Autodesk Inventor part; units mm, degrees
ref_plane "YZ Plane" through (0, 0, 0) normal (1, 0, 0) x (0, 1, 0)
ref_plane "XZ Plane" through (0, 0, 0) normal (0, 1, 0) x (-1, 0, 0)
ref_plane "XY Plane" through (0, 0, 0) normal (0, 0, 1) x (1, 0, 0)
sketch "Sketch1" plane through (0, 0, 0) normal (0, 1, 0) x (-1, 0, 0)
  line L0 (0, 0) -> (41.3, 0)
  line L1 (41.3, 0) -> (41.3, 41.3)
  line L2 (41.3, 41.3) -> (0, 41.3)
  line L3 (0, 41.3) -> (0, 0)
  dimension "d0" = 41.3
  dimension "d1" = 41.3
extrude "Extrusion1" add sketch "Sketch1" along normal blind 10
sketch "Sketch8" plane through (0, 10, 0) normal (0, 1, 0) x (1, 0, 0)
  line L0 (-1, -1) -> (-40.3, -1)
  line L1 (-40.3, -1) -> (-40.3, -40.3)
  line L2 (-40.3, -40.3) -> (-1, -40.3)
  line L3 (-1, -40.3) -> (-1, -1)
  line L4 (0, 0) -> (-41.3, 0)
  line L5 (0, -41.3) -> (0, 0)
  dimension "d61" = 39.3
  dimension "d62" = 39.3
  dimension "d63" = 1
  dimension "d64" = 1
extrude "Extrusion7" cut sketch "Sketch8" against normal blind 8.5
sketch "Sketch9" plane through (0, 1.5, 0) normal (0, 1, 0) x (1, 0, 0)
  line L0 (-3.45, -3.45) -> (-18.15, -3.45)
  line L1 (-18.15, -3.45) -> (-18.15, -18.15)
  line L2 (-18.15, -18.15) -> (-3.45, -18.15)
  line L3 (-3.45, -18.15) -> (-3.45, -3.45)
  line L4 (-1, -1) -> (-1, -40.3)
  line L5 (-40.3, -1) -> (-1, -1)
  line L6 (-23.15, -3.45) -> (-37.85, -3.45)
  line L7 (-37.85, -3.45) -> (-37.85, -18.15)
  line L8 (-37.85, -18.15) -> (-23.15, -18.15)
  line L9 (-23.15, -18.15) -> (-23.15, -3.45)
  line L10 (-23.15, -23.15) -> (-37.85, -23.15)
  line L11 (-37.85, -23.15) -> (-37.85, -37.85)
  line L12 (-37.85, -37.85) -> (-23.15, -37.85)
  line L13 (-23.15, -37.85) -> (-23.15, -23.15)
  line L14 (-40.3, -40.3) -> (-40.3, -1)
  line L15 (-18.15, -23.15) -> (-3.45, -23.15)
  line L16 (-3.45, -23.15) -> (-3.45, -37.85)
  line L17 (-3.45, -37.85) -> (-18.15, -37.85)
  line L18 (-18.15, -37.85) -> (-18.15, -23.15)
  point P0 (0, 0)
  dimension "d67" = 14.7
  dimension "d68" = 14.7
  dimension "d69" = 2.45
  dimension "d70" = 2.45
  dimension "d71" = 14.7
  dimension "d72" = 14.7
  dimension "d73" = 5
  dimension "d74" = 14.7
  dimension "d75" = 14.7
  dimension "d76" = 5
  dimension "d77" = 2.45
  dimension "d78" = 14.7
  dimension "d79" = 14.7
  dimension "d80" = 5
  dimension "d81" = 5
extrude "Extrusion8" cut sketch "Sketch9" against normal blind 8.5
properties part number "test plate"
Read the model definition and answer for the solid it produces. Units are mm, in the model's axes. A direction names the side the tool comes from. Give positions to 0.01 mm unless a question says otherwise; leave off trailing zeros. Write each loop counter-clockwise with the first axis right and the second up, starting at its lowest first coordinate (ties: lowest second). Pieces come first, ordered by that corner, then holes. Notation, with made-up numbers: (-36, 84) -> (23, 84) arc R14 cw to (23, 88) -> close; hole circle Ø6 at (17.5, -35.5). An arc over 180 degrees is marked (long way). Answer as a JSON object with one key per item and string values.
1) Straight lines are drawn through the part: probe 1 along X at (y, z) = (1, 25.5); probe 2 along Z at (x, y) = (-22, 9.5); probe 3 along X at (y, z) = (5.5, 33.5). For each, find the intervals that lie inside material, in ascending order. Write a range as from..to.
Findings below:
{"probe 1": "x = -41.3..-37.85, -23.15..-18.15, -3.45..0", "probe 2": "z = 0..1, 40.3..41.3", "probe 3": "x = -41.3..-40.3, -1..0"}
2) Section C-C on y = 5 is taken. Write down the section's boundary in (x, z), then the cut area to 3 significant figures.
Findings below:
{"outline": "(-41.3, 0) -> (0, 0) -> (0, 41.3) -> (-41.3, 41.3) -> close; hole (-40.3, 1) -> (-1, 1) -> (-1, 40.3) -> (-40.3, 40.3) -> close", "area": "161 mm^2"}
3) Section A-A on x = -9.5 is taken. Write down the section's boundary in (y, z), then the cut area to 4 significant figures.
Findings below:
{"outline": "(0, 0) -> (10, 0) -> (10, 1) -> (1.5, 1) -> (1.5, 3.45) -> (0, 3.45) -> close; (0, 18.15) -> (1.5, 18.15) -> (1.5, 23.15) -> (0, 23.15) -> close; (0, 37.85) -> (1.5, 37.85) -> (1.5, 40.3) -> (10, 40.3) -> (10, 41.3) -> (0, 41.3) -> close", "area": "34.85 mm^2"}
4) Section D-D on x = -21 is taken. Write down the section's boundary in (y, z), then the cut area to 4 significant figures.
Findings below:
{"outline": "(0, 0) -> (10, 0) -> (10, 1) -> (1.5, 1) -> (1.5, 40.3) -> (10, 40.3) -> (10, 41.3) -> (0, 41.3) -> close", "area": "78.95 mm^2"}
5) Section B-B on z = 13 is taken. Write down the section's boundary in (x, y).
Findings below:
{"outline": "(-41.3, 0) -> (-37.85, 0) -> (-37.85, 1.5) -> (-40.3, 1.5) -> (-40.3, 10) -> (-41.3, 10) -> close; (-23.15, 0) -> (-18.15, 0) -> (-18.15, 1.5) -> (-23.15, 1.5) -> close; (-3.45, 0) -> (0, 0) -> (0, 10) -> (-1, 10) -> (-1, 1.5) -> (-3.45, 1.5) -> close"}
6) A tool of negligible diameter and unlimited length cuts with its end or side. For faces 1 (the flat face through (-20, 5, 0)), 2 (the flat face through (-40.3, 6, 20)), 3 (the flat face through (-30, 1, 3.45)), from which of +Z, -Z, +X, -X, +Y, -Y can it reach the whole face along a straight path? Write none if from no direction.
Findings below:
{"face 1": "-Z, +X, -X, +Y, -Y", "face 2": "+Y", "face 3": "+Y, -Y"}
7) For a pull along X with two mould halves and no side action, classify faces 4 (the flat face through (-41.3, 5, 20)), 5 (the flat face through (-18.15, 1, 11)), 6 (the flat face through (-20, 0, 21)) as pulls with the +X half, pulls with the -X half, needs draft (parallel to the pull), parting line crosses it, or undercut.
Findings below:
{"face 4": "pulls with the -X half", "face 5": "undercut", "face 6": "needs draft"}
8) Flat-ended cylindrical pins translate along their axes: pin 1 Ø4 at (y, z) = (5.5, 21) entering from +X; pin 2 Ø8 at (x, z) = (-5.5, 6.5) entering from +Y. Find the tip coordinate at first contact, or state that the pin passes through.
Findings below:
{"pin 1": "stops at x = 0", "pin 2": "stops at y = 1.5"}
